```python
from build123d import *

# Parameters (mm, degrees)
SKETCH2_W           = 140
SKETCH2_H           = 164.092615239
BOSS_EXTRUDE1_DEPTH = 469.9
SHELL1_T            = 10
FILLET2_R           = 15
SKETCH4_R           = 44.25
CUT_EXTRUDE2_DEPTH  = 10


with BuildPart() as part:
    # Sketch2 → Boss-Extrude1 (new body)
    with BuildSketch(Plane(origin=(0, 0, 0), x_dir=(1, 0, 0), z_dir=(0, 1, 0))):
        with Locations((0, 12.04630762)):
            Rectangle(SKETCH2_W, SKETCH2_H)
    extrude(amount=-BOSS_EXTRUDE1_DEPTH)

    # Shell1
    shell1_openings = [part.faces().sort_by_distance(p)[0] for p in [
        (0, -469.9, -12.046307619),
    ]]
    offset(amount=SHELL1_T, openings=shell1_openings, kind=Kind.INTERSECTION)

    # Fillet2
    # the kernel refuses this fillet: 15 mm, written as the material it takes off along each edge
    with BuildSketch(Plane(origin=(65, -5, 65), x_dir=(0, 1, 0), z_dir=(1, 0, 0))) as fillet2_piece_1_section:
        Polygon((0, 0), (FILLET2_R, 0), (FILLET2_R, FILLET2_R), (0, FILLET2_R), align=None)
    fillet2_piece_1 = extrude(amount=FILLET2_R, mode=Mode.PRIVATE)
    fillet2_piece_1 = fillet2_piece_1 - Plane(origin=(65, -5, 65), x_dir=(0, -0.7071067811865475, -0.7071067811865475), z_dir=(1, 0, 0)) * Sphere(FILLET2_R, mode=Mode.PRIVATE)
    add(fillet2_piece_1, mode=Mode.SUBTRACT)
    with BuildSketch(Plane(origin=(-65, -5, 65), x_dir=(0, 0, 1), z_dir=(0, 1, 0))) as fillet2_piece_2_section:
        Polygon((0, 0), (FILLET2_R, 0), (FILLET2_R, -FILLET2_R), (0, -FILLET2_R), align=None)
    fillet2_piece_2 = extrude(amount=FILLET2_R, mode=Mode.PRIVATE)
    fillet2_piece_2 = fillet2_piece_2 - Plane(origin=(-65, -5, 65), x_dir=(0.7071067811865475, 0, -0.7071067811865475), z_dir=(0, 1, 0)) * Sphere(FILLET2_R, mode=Mode.PRIVATE)
    add(fillet2_piece_2, mode=Mode.SUBTRACT)
    with BuildSketch(Plane(origin=(-65, -5, -89.092615239), x_dir=(0, 1, 0), z_dir=(0, 0, -1))) as fillet2_piece_3_section:
        Polygon((0, 0), (FILLET2_R, 0), (FILLET2_R, -FILLET2_R), (0, -FILLET2_R), align=None)
    fillet2_piece_3 = extrude(amount=FILLET2_R, mode=Mode.PRIVATE)
    fillet2_piece_3 = fillet2_piece_3 - Plane(origin=(-65, -5, -89.092615239), x_dir=(0.7071067811865475, -0.7071067811865475, 0), z_dir=(0, 0, -1)) * Sphere(FILLET2_R, mode=Mode.PRIVATE)
    add(fillet2_piece_3, mode=Mode.SUBTRACT)
    with BuildSketch(Plane(origin=(65, -5, -89.092615239), x_dir=(1, 0, 0), z_dir=(0, 0, -1))) as fillet2_piece_4_section:
        Polygon((0, 0), (FILLET2_R, 0), (FILLET2_R, -FILLET2_R), (0, -FILLET2_R), align=None)
    fillet2_piece_4 = extrude(amount=FILLET2_R, mode=Mode.PRIVATE)
    fillet2_piece_4 = fillet2_piece_4 - Plane(origin=(65, -5, -89.092615239), x_dir=(-0.7071067811865475, -0.7071067811865475, 0), z_dir=(0, 0, -1)) * Sphere(FILLET2_R, mode=Mode.PRIVATE)
    add(fillet2_piece_4, mode=Mode.SUBTRACT)
    with BuildSketch(Plane(origin=(65, 10, 80), x_dir=(0, -1, 0), z_dir=(-1, 0, 0)), Plane(origin=(-65, 10, -104.092615239), x_dir=(0, -1, 0), z_dir=(1, 0, 0))) as fillet2_piece_5:
        with BuildLine():
            CenterArc((FILLET2_R, -FILLET2_R), FILLET2_R, 90, 90)
            Line((0, -FILLET2_R), (0, 0))
            Line((0, 0), (FILLET2_R, 0))
        make_face()
    extrude(amount=130, mode=Mode.SUBTRACT)
    with BuildSketch(Plane(origin=(-80, 10, 65), x_dir=(0, -1, 0), z_dir=(0, 0, -1)), Plane(origin=(80, 10, -89.092615239), x_dir=(0, -1, 0), z_dir=(0, 0, 1))) as fillet2_piece_6:
        with BuildLine():
            CenterArc((FILLET2_R, -FILLET2_R), FILLET2_R, 90, 90)
            Line((0, -FILLET2_R), (0, 0))
            Line((0, 0), (FILLET2_R, 0))
        make_face()
    extrude(amount=154.092615239, mode=Mode.SUBTRACT)
    with BuildSketch(Plane(origin=(80, -507.4, 80), x_dir=(-1, 0, 0), z_dir=(0, 1, 0)), Plane(origin=(-80, -5, 80), x_dir=(1, 0, 0), z_dir=(0, -1, 0)), Plane(origin=(-80, -5, -104.092615239), x_dir=(0, 0, 1), z_dir=(0, -1, 0)), Plane(origin=(80, -5, -104.092615239), x_dir=(-1, 0, 0), z_dir=(0, -1, 0))) as fillet2_piece_7:
        with BuildLine():
            CenterArc((FILLET2_R, -FILLET2_R), FILLET2_R, 90, 90)
            Line((0, -FILLET2_R), (0, 0))
            Line((0, 0), (FILLET2_R, 0))
        make_face()
    extrude(amount=502.4, mode=Mode.SUBTRACT)

    # Sketch4 → Cut-Extrude2 (cut)
    with BuildSketch(Plane(origin=(44.675144213, 0, 80), x_dir=(-1, 0, 0), z_dir=(0, 0, -1))):
        with Locations((44.675144213, -55)):
            Circle(SKETCH4_R)
    extrude(amount=CUT_EXTRUDE2_DEPTH, mode=Mode.SUBTRACT)


solid = part.part
```
Verification items for the finished model (mm, model axes). A direction names the side the tool comes from. Give positions to 0.01 mm unless a question says otherwise; leave off trailing zeros. Loops run counter-clockwise (first coordinate to the right, second up) from the corner with the lowest first, then second, coordinate; pieces in that order, holes last. Notation, with made-up numbers: M 87,78 L 106,78 A6 cw 106,86 Z; hole C 18,-13 d2. An arc over 180 degrees is marked long. Return JSON: item names as keys, results as strings.
1) Section check D-D, the plane x = -53. Enter the section's corners in (y, z).
Findings:
{"outline": "M -469.9,-104.09 L -5,-104.09 A15 ccw 10,-89.09 L 10,65 A15 ccw -5,80 L -469.9,80 L -469.9,70 L 0,70 L 0,-94.09 L -469.9,-94.09 Z"}
2) Section check A-A, the plane x = 0. Enter the section's corners in (y, z), and give its area (3 significant figures).
Findings:
{"outline": "M -469.9,-104.09 L -5,-104.09 A15 ccw 10,-89.09 L 10,65 A15 ccw -5,80 L -10.75,80 L -10.75,70 L 0,70 L 0,-94.09 L -469.9,-94.09 Z; M -469.9,70 L -99.25,70 L -99.25,80 L -469.9,80 Z", "area": "10,300 mm2"}
3) Section check C-C, the plane z = 16.5. Enter the section's corners in (x, y).
Findings:
{"outline": "M -80,-469.9 L -70,-469.9 L -70,0 L 70,0 L 70,-469.9 L 80,-469.9 L 80,-5 A15 ccw 65,10 L -65,10 A15 ccw -80,-5 Z"}
4) Gauge pin test, flat end, axial feed: P1, Ø6, axis at x = 26, z = -70.5, coming from the -Y side. Record the tip position at first contact, or that the pin passes through.
Findings:
{"P1": "stops at y = 0"}
5) Material ranges on L1, parallel to X at y = -424.5, z = 15; L2, parallel to Z at x = -40, y = -101; L3, parallel to X at y = -142, z = -90.5, recorded low to high. Write a range as [from, to].
Findings:
{"L1": "x = [-80, -70], [70, 80]", "L2": "z = [-104.09, -94.09], [70, 80]", "L3": "x = [-79.93, -70], [70, 79.93]"}
6) Section check B-B, the plane y = -296.5. Enter the section's corners in (x, z), and give its area (3 significant figures).
Findings:
{"outline": "M -80,-89.09 A15 ccw -65,-104.09 L 65,-104.09 A15 ccw 80,-89.09 L 80,65 A15 ccw 65,80 L -65,80 A15 ccw -80,65 Z; hole M -70,-94.09 L 70,-94.09 L 70,70 L -70,70 Z", "area": "6,290 mm2"}
7) Tool access check on faces 1 (the flat face through (-1, 0, -13)), 2 (the cylindrical face through (-0.91, 5.489, -99.815)), 3 (the cylindrical face through (5.76, -11.127, 75.07)). Record the directions out of +Z, -Z, +X, -X, +Y, -Y that give a thin tool (end or side, any length) a straight path to the whole face; none if there is none.
Findings:
{"face 1": "-Y", "face 2": "-Z, +X, -X, +Y", "face 3": "+Z"}
8) Mould release check, pull along Z, two halves, no side actions. Record for faces 4 (the flat face through (-1, -234, -104.093)), 5 (the cylindrical face through (75.49, -240.7, 75.72)), 6 (the flat face through (80, -234, -11)), 7 (the flat face through (70, -232, -11)): released by +Z, released by -Z, zero draft, split by the parting line, or undercut.
Findings:
{"face 4": "released by -Z", "face 5": "released by +Z", "face 6": "zero draft", "face 7": "undercut"}
